For this review, take the finished solid that the model builds, in its own axes (mm). A direction names the side the tool comes from. Give positions to 0.01 mm unless a question says otherwise; leave off trailing zeros. Loops run counter-clockwise (first coordinate to the right, second up) from the corner with the lowest first, then second, coordinate; pieces in that order, holes last. Notation, with made-up numbers: (16.25, 3.25) -> (65.25, 3.25) arc R13 ccw to (65.25, 28.25) -> close; hole circle Ø1 at (71, 49). An arc over 180 degrees is marked (long way). One line per question, with ' | ' between items. Start each with the question number.
(1) Draft analysis for pull direction Y (two halves, no side actions). For faces 1 (the cylindrical face through (-78.797, -53.859, 12.325)), 2 (the flat face through (0, 44, 25)), 3 (the cylindrical face through (75.923, -48.226, 12.325)), state which applies: +Y half, -Y half, draft (parallel to the pull), parting line (faces both ways), or undercut.
(2) Consider section D-D (x = 57). Write out the cut boundary in (y, z).
(3) Consider section B-B (y = -7.5). Write out the cut boundary in (x, z), and give its area (3 significant figures).
(4) Consider section A-A (x = -49.5). Write out the cut boundary in (y, z), and give its area (3 significant figures).
(5) Tool access review of faces 4 (the cylindrical face through (59.296, 37.889, 4.211)), 5 (the flat face through (0, 49, 25)), 6 (the flat face through (1, -33.25, 3)): name each direction out of +Z, -Z, +X, -X, +Y, -Y from which nothing blocks a thin tool from reaching the whole face with its end or side.
(6) Insertion check: P1, Ø2.5, axis at x = 75, y = -50, coming from the +Z side. The pin has a flat end and moves straight along its axis. Give the tip position at first contact, or say it passes through.
(7) Wall thickness on probe 1 along Y at (x, z) = (-75, 15); probe 2 along Y at (x, z) = (32, 4); probe 3 along X at (y, z) = (25, 18): over which ranges is each line inside the solid? List them lowest first.
(8) Consider section C-C (z = 7). Write out the cut boundary in (x, y).
Autodesk Fusion 360 part; units mm, degrees
sketch "Sketch1" plane through (0, 0, 0) normal (0, 0, 1) x (1, 0, 0)
  line L0 (76, -55) -> (-76, -55)
  line L1 (-80, -51) -> (-80, 51)
  line L2 (-76, 55) -> (76, 55)
  line L3 (80, 51) -> (80, -51)
  line L4 (80, -55) -> (-80, 55) construction
  line L5 (-80, -55) -> (80, 55) construction
  arc A0 (-76, 55) -> (-80, 51) centre (-76, 51) ccw
  arc A1 (80, 51) -> (76, 55) centre (76, 51) ccw
  arc A2 (76, -55) -> (80, -51) centre (76, -51) ccw
  arc A3 (-80, -51) -> (-76, -55) centre (-76, -51) ccw
  circle A4 centre (-75, 50) radius 2
  line L6 (0, 55) -> (0, -55) construction
  line L7 (80, 0) -> (-80, 0) construction
  circle A5 centre (75, 50) radius 2
  circle A6 centre (75, -50) radius 2
  circle A7 centre (-75, -50) radius 2
  dimension "d1" = 160
  dimension "d2" = 110
  dimension "d26" = 4
  dimension "d27" = 4
  dimension "d28" = 4
  dimension "d29" = 4
  dimension "d30" = 4
  dimension "d31" = 5
  dimension "d32" = 5
extrude "Extrude1" add sketch "Sketch1" along normal blind 25
sketch "Sketch2" plane through (0, 0, 25) normal (0, 0, 1) x (-1, 0, 0)
  line L0 (-76, -55) -> (76, -55)
  line L1 (80, -51) -> (80, 51)
  line L2 (76, 55) -> (-76, 55)
  line L3 (-80, 51) -> (-80, -51)
  line L4 (-64.4, 43.25) -> (64.4, 43.25)
  line L5 (64.4, 43.25) -> (64.4, -43.25)
  line L6 (64.4, -43.25) -> (-64.4, -43.25)
  line L7 (-64.4, -43.25) -> (-64.4, 43.25)
  line L8 (-64.4, 43.25) -> (64.4, -43.25) construction
  line L9 (64.4, 43.25) -> (-64.4, -43.25) construction
  arc A0 (76, -55) -> (80, -51) centre (76, -51) ccw
  arc A1 (80, 51) -> (76, 55) centre (76, 51) ccw
  arc A2 (-76, 55) -> (-80, 51) centre (-76, 51) ccw
  arc A3 (-80, -51) -> (-76, -55) centre (-76, -51) ccw
  circle A4 centre (75, 50) radius 2
  circle A5 centre (-75, 50) radius 2
  circle A6 centre (-75, -50) radius 2
  circle A7 centre (75, -50) radius 2
  dimension "d5" = 128.8
  dimension "d6" = 86.5
extrude "Extrude2" cut sketch "Sketch2" against normal blind 20 contours L4 L5 L6 L7
sketch "Sketch3" plane through (0, 0, 25) normal (0, 0, 1) x (-1, 0, 0)
  line L0 (64.4, 43.25) -> (64.4, -43.25)
  line L1 (64.4, -43.25) -> (-64.4, -43.25)
  line L2 (-64.4, -43.25) -> (-64.4, 43.25)
  line L3 (-64.4, 43.25) -> (64.4, 43.25)
  line L4 (-76, -55) -> (76, -55)
  line L5 (80, -51) -> (80, 51)
  line L6 (76, 55) -> (-76, 55)
  line L7 (-80, 51) -> (-80, -51)
  line L8 (-72.0964, 47.0964) -> (72.0964, 47.0964) construction
  line L9 (72.0964, 47.0964) -> (72.0964, -47.0964) construction
  line L10 (72.0964, -47.0964) -> (-72.0964, -47.0964) construction
  line L11 (-72.0964, -47.0964) -> (-72.0964, 47.0964) construction
  line L12 (-72.0964, 47.0964) -> (72.0964, -47.0964) construction
  line L13 (72.0964, 47.0964) -> (-72.0964, -47.0964) construction
  line L14 (70.6619, 35.3929) -> (70.6619, -35.3929)
  line L15 (60.3929, -45.6619) -> (-60.3929, -45.6619)
  line L16 (-70.6619, -35.3929) -> (-70.6619, 35.3929)
  line L17 (-70.6619, 45.6619) -> (70.6619, -45.6619) construction
  line L18 (70.6619, 45.6619) -> (-70.6619, -45.6619) construction
  line L19 (-60.3929, 48.5309) -> (60.3929, 48.5309)
  line L20 (73.5309, 35.3929) -> (73.5309, -35.3929)
  line L21 (60.3929, -48.5309) -> (-60.3929, -48.5309)
  line L22 (-73.5309, -35.3929) -> (-73.5309, 35.3929)
  line L23 (-73.5309, 48.5309) -> (73.5309, -48.5309) construction
  line L24 (73.5309, 48.5309) -> (-73.5309, -48.5309) construction
  arc A0 (60.3929, -45.6619) -> (70.6619, -35.3929) centre (60.3929, -35.3929) ccw
  arc A1 (60.3929, -48.5309) -> (73.5309, -35.3929) centre (60.3929, -35.3929) ccw
  line L25 (0, -55) -> (0, 55) construction
  line L26 (-80, 0) -> (80, 0) construction
  arc A2 (-70.6619, -35.3929) -> (-60.3929, -45.6619) centre (-60.3929, -35.3929) ccw
  arc A3 (-73.5309, -35.3929) -> (-60.3929, -48.5309) centre (-60.3929, -35.3929) ccw
  arc A4 (-60.3929, 45.6619) -> (-70.6619, 35.3929) centre (-60.3929, 35.3929) ccw
  arc A5 (-60.3929, 48.5309) -> (-73.5309, 35.3929) centre (-60.3929, 35.3929) ccw
  arc A6 (70.6619, 35.3929) -> (60.3929, 45.6619) centre (60.3929, 35.3929) ccw
  arc A7 (73.5309, 35.3929) -> (60.3929, 48.5309) centre (60.3929, 35.3929) ccw
  line L27 (-60.3929, 45.6619) -> (60.3929, 45.6619)
  arc A8 (76, -55) -> (80, -51) centre (76, -51) ccw
  arc A9 (80, 51) -> (76, 55) centre (76, 51) ccw
  arc A10 (-76, 55) -> (-80, 51) centre (-76, 51) ccw
  arc A11 (-80, -51) -> (-76, -55) centre (-76, -51) ccw
  circle A12 centre (75, 50) radius 2
  circle A13 centre (-75, 50) radius 2
  circle A14 centre (-75, -50) radius 2
  circle A15 centre (75, -50) radius 2
  dimension "d9" = 144.1928
  dimension "d15" = 94.1928
  dimension "d16" = 1.4345
  dimension "d17" = 1.4345
  dimension "d18" = 1.4345
  dimension "d19" = 1.4345
  dimension "d20" = 10.269
  dimension "d21" = 13.138
extrude "Extrude3" cut sketch "Sketch3" against normal blind 1.424 contours L19 L20 L21 L22 A1 A3 A5 A7
draft "Draft1" angle 10 neutral plane through (0, 0, 23.576) pull (0, 0, 1) 16 faces at (-70.6619, -11.7976, 24.5253) (-67.8249, 42.4793, 24.0507) (-20.131, 45.6619, 24.5253) (67.4793, 42.8249, 24.0507) (70.6619, 11.7976, 24.5253) (67.8249, -42.4793, 24.0507) (20.131, -45.6619, 24.5253) (-64.2095, -44.9263, 24.5253) (-73.5309, -11.7976, 24.5253) (-70.7201, -43.5143, 24.0507) (20.131, -48.5309, 24.5253) (68.5143, -45.7201, 24.0507) (73.5309, 11.7976, 24.5253) (70.7201, 43.5143, 24.0507) (-20.131, 48.5309, 24.5253) (-71.0948, 43.0137, 24.0507)
sketch "Sketch4" plane through (0, 0, 5) normal (0, 0, 1) x (-1, 0, 0)
  line L0 (-64.4, -43.25) -> (64.4, -43.25)
  line L1 (64.4, -43.25) -> (64.4, 43.25)
  line L2 (64.4, 43.25) -> (-64.4, 43.25)
  line L3 (-64.4, 43.25) -> (-64.4, -43.25)
  line L4 (-54.4, 33.25) -> (54.4, 33.25)
  line L5 (54.4, 33.25) -> (54.4, -33.25)
  line L6 (54.4, -33.25) -> (-54.4, -33.25)
  line L7 (-54.4, -33.25) -> (-54.4, 33.25)
  line L8 (-54.4, 33.25) -> (54.4, -33.25) construction
  line L9 (54.4, 33.25) -> (-54.4, -33.25) construction
  dimension "d35" = 10
  dimension "d36" = 10
extrude "Extrude4" cut sketch "Sketch4" against normal blind 5 contours L4 L5 L6 L7
sketch "Sketch5" plane through (0, 0, 5) normal (0, 0, 1) x (-1, 0, 0)
  line L0 (54.4, 33.25) -> (54.4, -33.25)
  line L1 (54.4, -33.25) -> (-54.4, -33.25)
  line L2 (-54.4, -33.25) -> (-54.4, 33.25)
  line L3 (-54.4, 33.25) -> (54.4, 33.25)
  line L4 (-64.4, -43.25) -> (64.4, -43.25)
  line L5 (64.4, -43.25) -> (64.4, 43.25)
  line L6 (64.4, 43.25) -> (-64.4, 43.25)
  line L7 (-64.4, 43.25) -> (-64.4, -43.25)
  line L8 (-60.8342, 39.6842) -> (60.8342, 39.6842) construction
  line L9 (60.8342, 39.6842) -> (60.8342, -39.6842) construction
  line L10 (60.8342, -39.6842) -> (-60.8342, -39.6842) construction
  line L11 (-60.8342, -39.6842) -> (-60.8342, 39.6842) construction
  line L12 (-60.8342, 39.6842) -> (60.8342, -39.6842) construction
  line L13 (60.8342, 39.6842) -> (-60.8342, -39.6842) construction
  line L14 (59.7842, 31.4252) -> (59.7842, -31.4252)
  line L15 (52.5752, -38.6342) -> (-52.5752, -38.6342)
  line L16 (-59.7842, -31.4252) -> (-59.7842, 31.4252)
  line L17 (-57.1085, 36.9051) -> (59.7842, -38.6342) construction
  line L18 (57.4574, 36.3074) -> (-57.4574, -36.3074) construction
  line L19 (-52.8062, 40.6187) -> (52.8062, 40.6187)
  line L20 (61.8842, 31.5407) -> (61.8842, -31.5407)
  line L21 (52.8062, -40.6187) -> (-52.8062, -40.6187)
  line L22 (-61.8842, -31.5407) -> (-61.8842, 31.5407)
  line L23 (-58.9962, 38.7231) -> (61.8842, -40.6187) construction
  line L24 (59.3264, 38.1764) -> (-59.3264, -38.1764) construction
  arc A0 (52.5752, -38.6342) -> (59.7842, -31.4252) centre (52.5752, -31.4252) ccw
  arc A1 (52.8062, -40.6187) -> (61.8842, -31.5407) centre (52.8062, -31.5407) ccw
  line L25 (0, -43.25) -> (0, 43.25) construction
  line L26 (-64.4, 0) -> (64.4, 0) construction
  arc A2 (-59.7842, -31.4252) -> (-52.5752, -38.6342) centre (-52.5752, -31.4252) ccw
  arc A3 (-61.8842, -31.5407) -> (-52.8062, -40.6187) centre (-52.8062, -31.5407) ccw
  arc A4 (59.7842, 31.4252) -> (52.5752, 38.6342) centre (52.5752, 31.4252) ccw
  arc A5 (61.8842, 31.5407) -> (52.8062, 40.6187) centre (52.8062, 31.5407) ccw
  arc A6 (-52.5752, 38.6342) -> (-59.7842, 31.4252) centre (-52.5752, 31.4252) ccw
  arc A7 (-52.8062, 40.6187) -> (-61.8842, 31.5407) centre (-52.8062, 31.5407) ccw
  line L27 (-52.5752, 38.6342) -> (52.5752, 38.6342)
  dimension "d42" = 121.6684
  dimension "d43" = 79.3684
  dimension "d44" = 1.05
  dimension "d45" = 0.9345
  dimension "d46" = 1.05
  dimension "d47" = 1.05
  dimension "d48" = 7.209
  dimension "d49" = 9.078
extrude "Extrude5" cut sketch "Sketch5" against normal blind 1.6 contours L19 L20 L21 L22 A1 A3 A5 A7
equation "d9 = ( ORingPerimeter - 100 mm ) / 4 + 50 mm"
equation "ORingDiameter = 1.78 mm"
equation "ORingInnerDiameter = 150 mm"
equation "ORingPerimeter = 2 * 3.1412 * ( ( ORingInnerDiameter / 2 ) + ORingDiameter / 2 )"
equation "PanelWidth = 80 mm"
equation "PanelLength = 115 mm"
equation "d15 = ( ORingPerimeter - 100 mm ) / 4"
equation "d16 = ( ( ORingDiameter * 1.05 ) / 2 ) + 0.5 mm"
equation "d17 = ( ( ORingDiameter * 1.05 ) / 2 ) + 0.5 mm"
equation "d18 = ( ( ORingDiameter * 1.05 ) / 2 ) + 0.5 mm"
equation "d19 = ( ( ORingDiameter * 1.05 ) / 2 ) + 0.5 mm"
equation "d20 = ( ORingDiameter ) * 6 + ORingDiameter * 0.05 - 0.5 mm"
equation "d21 = ( ORingDiameter ) * 6 + ( ORingDiameter * 1.1 ) + 0.5 mm"
equation "d22 = -ORingDiameter * 0.8"
equation "ORing2Diameter = 2 mm"
equation "ORing2InnerDiameter = 126 mm"
equation "ORing2Perimeter = 2 * 3.1412 * ( ( ORing2InnerDiameter / 2 ) + ORing2Diameter / 2 )"
equation "d42 = ( ORing2Perimeter - 84.6 mm ) / 4 + 42.3 mm"
equation "d43 = ( ORing2Perimeter - 84.6 mm ) / 4"
equation "d44 = ( ORing2Diameter * 1.05 ) / 2"
equation "d45 = ( ORingDiameter * 1.05 ) / 2"
equation "d46 = ( ORing2Diameter * 1.05 ) / 2"
equation "d47 = ( ORing2Diameter * 1.05 ) / 2"
equation "d48 = ( ORingDiameter ) * 4 + ORingDiameter * 0.05 - 0.0 mm"
equation "d49 = ( ORingDiameter ) * 4 + ORingDiameter * 1.1 + 0 mm"
equation "d50 = -ORing2Diameter * 0.8"
A:
1) face 1: -Y half | face 2: draft | face 3: undercut
2) outline: (-55, 0) -> (55, 0) -> (55, 25) -> (48.78, 25) -> (48.53, 23.58) -> (45.66, 23.58) -> (45.41, 25) -> (43.25, 25) -> (43.25, 5) -> (39.59, 5) -> (39.59, 3.4) -> (37.12, 3.4) -> (37.12, 5) -> (-37.12, 5) -> (-37.12, 3.4) -> (-39.59, 3.4) -> (-39.59, 5) -> (-43.25, 5) -> (-43.25, 25) -> (-45.41, 25) -> (-45.66, 23.58) -> (-48.53, 23.58) -> (-48.78, 25) -> (-55, 25) -> close
3) outline: (-80, 0) -> (-54.4, 0) -> (-54.4, 5) -> (-59.78, 5) -> (-59.78, 3.4) -> (-61.88, 3.4) -> (-61.88, 5) -> (-64.4, 5) -> (-64.4, 25) -> (-70.41, 25) -> (-70.66, 23.58) -> (-73.53, 23.58) -> (-73.78, 25) -> (-80, 25) -> close; (54.4, 0) -> (80, 0) -> (80, 25) -> (73.78, 25) -> (73.53, 23.58) -> (70.66, 23.58) -> (70.41, 25) -> (64.4, 25) -> (64.4, 5) -> (61.88, 5) -> (61.88, 3.4) -> (59.78, 3.4) -> (59.78, 5) -> (54.4, 5) -> close | area: 864 mm^2
4) outline: (-55, 0) -> (-33.25, 0) -> (-33.25, 5) -> (-38.63, 5) -> (-38.63, 3.4) -> (-40.62, 3.4) -> (-40.62, 5) -> (-43.25, 5) -> (-43.25, 25) -> (-45.41, 25) -> (-45.66, 23.58) -> (-48.53, 23.58) -> (-48.78, 25) -> (-55, 25) -> close; (33.25, 0) -> (55, 0) -> (55, 25) -> (48.78, 25) -> (48.53, 23.58) -> (45.66, 23.58) -> (45.41, 25) -> (43.25, 25) -> (43.25, 5) -> (40.62, 5) -> (40.62, 3.4) -> (38.63, 3.4) -> (38.63, 5) -> (33.25, 5) -> close | area: 672 mm^2
5) face 4: +Z | face 5: +Z, +X, -X, +Y, -Y | face 6: +Z, -Z
6) P1: passes through
7) probe 1: y = -55 to -52, -48 to 48, 52 to 55 | probe 2: y = -55 to -40.62, -38.63 to -33.25, 33.25 to 38.63, 40.62 to 55 | probe 3: x = -80 to -64.4, 64.4 to 80
8) outline: (-80, -51) arc R4 ccw to (-76, -55) -> (76, -55) arc R4 ccw to (80, -51) -> (80, 51) arc R4 ccw to (76, 55) -> (-76, 55) arc R4 ccw to (-80, 51) -> close; hole circle Ø4 at (-75, -50); hole circle Ø4 at (-75, 50); hole (-64.4, -43.25) -> (64.4, -43.25) -> (64.4, 43.25) -> (-64.4, 43.25) -> close; hole circle Ø4 at (75, -50); hole circle Ø4 at (75, 50)
